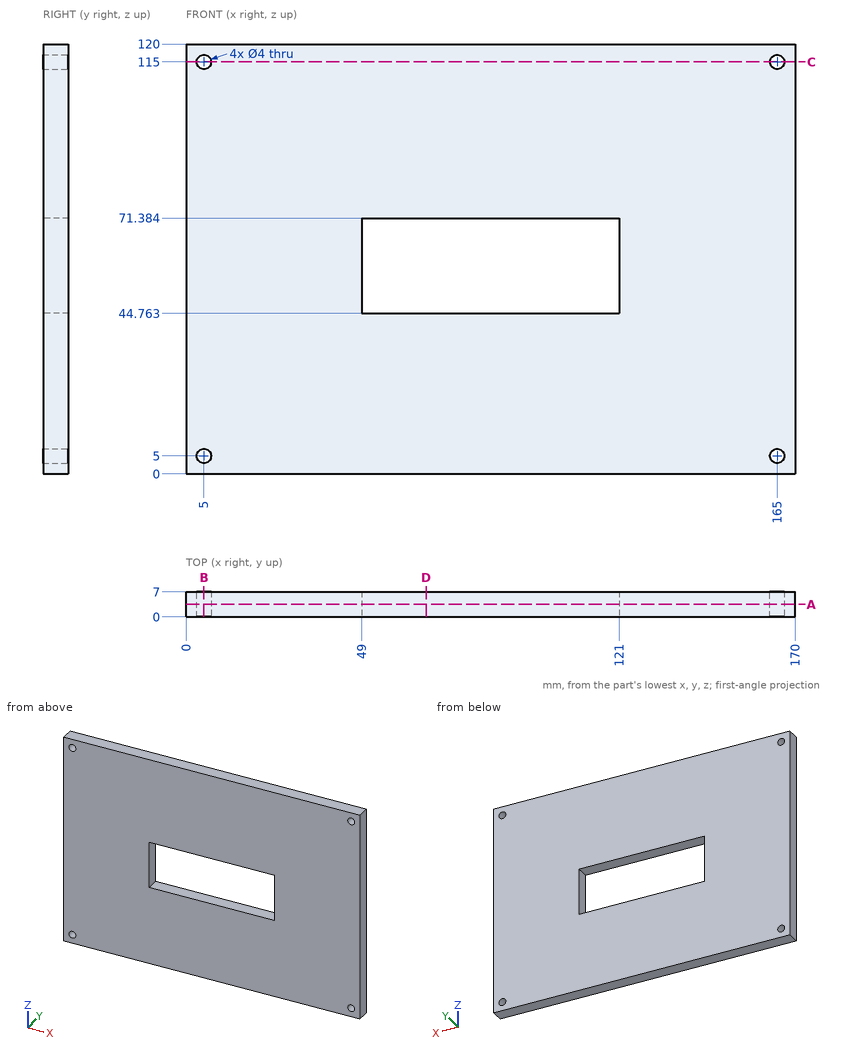
Can you work these out from the drawing? Everything is in mm from the part's minimum corner. Give positions to 0.01 mm unless a question says otherwise; leave off trailing zeros. Order: outer loops, then holes, each group sorted by start corner. A loop starts at its lowest first (then second) coordinate and runs counter-clockwise, first axis right, second up.
1. Suppose I cut it at D-D (x = 67). List the corners of the cut face in (y, z) for me, plus the area to 3 significant figures.
2. I need wall thicknesses on L1, parallel to X at y = 2.75, z = 115; L2, parallel to Z at x = 5, y = 2; L3, parallel to Z at x = 91, y = 6.5. Which ranges of each line are inside material? Lowest first, please.
3. Suppose I cut it at A-A (y = 3.5). List the corners of the cut face in (x, z) for me, plus the area to 3 significant figures.
4. Will this pin go through, and if not, where does the flat tip stop? P1, Ø5, axis at x = 5, z = 5, coming from the -Y side.
5. Suppose I cut it at C-C (z = 115). List the corners of the cut face in (x, y) for me, plus the area to 3 significant figures.
6. Suppose I cut it at B-B (x = 5). List the corners of the cut face in (y, z) for me.
Solved:
1. outline: (0, 0) - (7, 0) - (7, 44.76) - (0, 44.76) - close; (0, 71.38) - (7, 71.38) - (7, 120) - (0, 120) - close
1. area: 654 mm2
2. L1: x = 0 to 3, 7 to 163, 167 to 170
2. L2: z = 0 to 3, 7 to 113, 117 to 120
2. L3: z = 0 to 44.76, 71.38 to 120
3. outline: (0, 0) - (170, 0) - (170, 120) - (0, 120) - close; hole circle Ø4 at (5, 5); hole circle Ø4 at (5, 115); hole (49, 44.76) - (121, 44.76) - (121, 71.38) - (49, 71.38) - close; hole circle Ø4 at (165, 5); hole circle Ø4 at (165, 115)
3. area: 18,400 mm2
4. P1: stops at y = 0
5. outline: (0, 0) - (3, 0) - (3, 7) - (0, 7) - close; (7, 0) - (163, 0) - (163, 7) - (7, 7) - close; (167, 0) - (170, 0) - (170, 7) - (167, 7) - close
5. area: 1,130 mm2
6. outline: (0, 0) - (7, 0) - (7, 3) - (0, 3) - close; (0, 7) - (7, 7) - (7, 113) - (0, 113) - close; (0, 117) - (7, 117) - (7, 120) - (0, 120) - close
